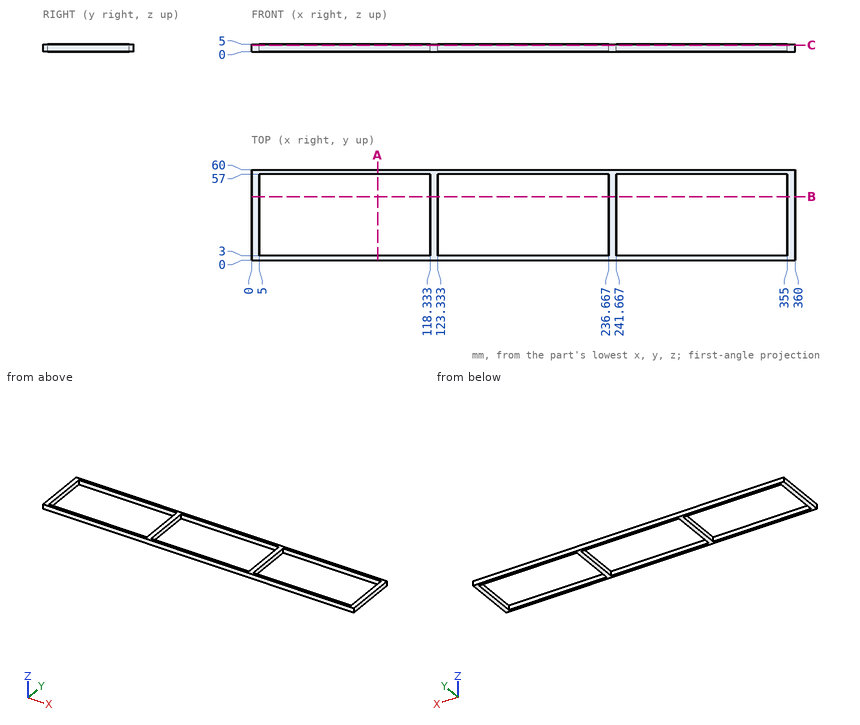
Verification items for this drawing (mm, ordinates from the low corner). Give positions to 0.01 mm unless a question says otherwise; leave off trailing zeros. Loops run counter-clockwise (first coordinate to the right, second up) from the corner with the lowest first, then second, coordinate; pieces in that order, holes last. Notation, with made-up numbers: M 76,17.25 L 126,17.25 A17 cw 126,42.25 Z; hole C -6,12.25 d1. An arc over 180 degrees is marked long. Return JSON: item names as keys, results as strings. Group by question number.
1. Go/stop test with flat-tipped pins: pin 1 (2.5 mm diameter, centred on y = 22, z = 1.5, fed in from -X); pin 2 (12 mm diameter, centred on x = 286, y = 45.5, fed in from +Z). Record where each tip stops, or that it passes through.
2. Cross-section at A-A on x = 83.5. Record the boundary of the cut face in (y, z).
3. Cross-section at C-C on z = 4.2. Record the boundary of the cut face in (x, y), plus the area to 3 significant figures.
4. Cross-section at B-B on y = 42. Record the boundary of the cut face in (x, z), plus the area to 3 significant figures.
5. Thickness scan on L1, parallel to X at y = 38, z = 3; L2, parallel to Y at x = 285, z = 4. Record the ranges inside material, lowest first.
Return value:
{
 "1": {"pin 1": "x = 0", "pin 2": "through"},
 "2": {"outline": "M 0,0 L 3,0 L 3,5 L 0,5 Z; M 57,0 L 60,0 L 60,5 L 57,5 Z"},
 "3": {"outline": "M 0,0 L 360,0 L 360,60 L 0,60 Z; hole M 5,3 L 118.33,3 L 118.33,57 L 5,57 Z; hole M 123.33,3 L 236.67,3 L 236.67,57 L 123.33,57 Z; hole M 241.67,3 L 355,3 L 355,57 L 241.67,57 Z", "area": "3,240 mm^2"},
 "4": {"outline": "M 0,0 L 5,0 L 5,5 L 0,5 Z; M 118.33,0 L 123.33,0 L 123.33,5 L 118.33,5 Z; M 236.67,0 L 241.67,0 L 241.67,5 L 236.67,5 Z; M 355,0 L 360,0 L 360,5 L 355,5 Z", "area": "100 mm^2"},
 "5": {"L1": "0 to 5, 118.33 to 123.33, 236.67 to 241.67, 355 to 360", "L2": "0 to 3, 57 to 60"}
}
